from build123d import *

# Parameters (mm, degrees)
F0_R     = 4.175
F0_W     = 52
F0_H     = 52
F0_W_2   = 7
F0_W_3   = 5
F0_H_2   = 50
F0_R_2   = 3.175
F1_DEPTH = 2.5
F2_DEPTH = 10
F3_DEPTH = 10
F4_DEPTH = 10


with BuildPart() as f1:
    # F0 (on Top) → F1 (new body)
    with BuildSketch(Plane.XY):
        with BuildLine():
            Line((-84, -30), (84, -30))
            ThreePointArc((84, -30), (88.2426406871, -28.2426406871), (90, -24))
            Line((90, -24), (90, 24))
            ThreePointArc((90, 24), (88.2426406871, 28.2426406871), (84, 30))
            Line((84, 30), (-84, 30))
            ThreePointArc((-84, 30), (-88.2426406871, 28.2426406871), (-90, 24))
            Line((-90, 24), (-90, -24))
            ThreePointArc((-90, -24), (-88.2426406871, -28.2426406871), (-84, -30))
        make_face()
        with BuildLine():
            ThreePointArc((89, -23), (87.2426406871, -27.2426406871), (83, -29))
            Line((83, -29), (-83, -29))
            ThreePointArc((-83, -29), (-87.2426406871, -27.2426406871), (-89, -23))
            Line((-89, -23), (-89, 23))
            ThreePointArc((-89, 23), (-87.2426406871, 27.2426406871), (-83, 29))
            Line((-83, 29), (83, 29))
            ThreePointArc((83, 29), (87.2426406871, 27.2426406871), (89, 23))
            Line((89, 23), (89, -23))
        make_face(mode=Mode.SUBTRACT)
        with BuildLine():
            Line((-83, -29), (83, -29))
            ThreePointArc((83, -29), (87.2426406871, -27.2426406871), (89, -23))
            Line((89, -23), (89, 23))
            ThreePointArc((89, 23), (87.2426406871, 27.2426406871), (83, 29))
            Line((83, 29), (-83, 29))
            ThreePointArc((-83, 29), (-87.2426406871, 27.2426406871), (-89, 23))
            Line((-89, 23), (-89, -23))
            ThreePointArc((-89, -23), (-87.2426406871, -27.2426406871), (-83, -29))
        make_face()
        with Locations((-82, 0)):
            Circle(F0_R, mode=Mode.SUBTRACT)
        with Locations((-45, 0)):
            Rectangle(F0_W, F0_H, mode=Mode.SUBTRACT)
        with Locations((70, 0)):
            Rectangle(F0_W_2, F0_H, mode=Mode.SUBTRACT)
        with Locations((-45, 0)):
            Rectangle(F0_W, F0_H)
        Polygon((-20, 0), (-20, -25), (-45, -25), (-70, -25), (-70, 0), (-70, 25), (-45, 25), (-20, 25), align=None, mode=Mode.SUBTRACT)
        with Locations((70, 0)):
            Rectangle(F0_W_2, F0_H)
        with Locations((70, 0)):
            Rectangle(F0_W_3, F0_H_2, mode=Mode.SUBTRACT)
        with Locations((70, 0)):
            Rectangle(F0_W_3, F0_H_2)
        with BuildLine():
            Line((-45, -25), (-20, -25))
            Line((-20, -25), (-20, 0))
            ThreePointArc((-20, 0), (-27.3223304703, -17.6776695297), (-45, -25))
        make_face()
        with BuildLine():
            ThreePointArc((-45, 25), (-27.3223304703, 17.6776695297), (-20, 0))
            Line((-20, 0), (-20, 25))
            Line((-20, 25), (-45, 25))
        make_face()
        with BuildLine():
            Line((-70, 25), (-70, 0))
            ThreePointArc((-70, 0), (-62.6776695297, 17.6776695297), (-45, 25))
            Line((-45, 25), (-70, 25))
        make_face()
        with BuildLine():
            Line((-70, -25), (-45, -25))
            ThreePointArc((-45, -25), (-62.6776695297, -17.6776695297), (-70, 0))
            Line((-70, 0), (-70, -25))
        make_face()
        with Locations((-82, 0)):
            Circle(F0_R)
        with Locations((-82, 0)):
            Circle(F0_R_2, mode=Mode.SUBTRACT)
        with Locations((-82, 0)):
            Circle(F0_R_2)
    extrude(amount=F1_DEPTH)

    # F0 (on Top) → F2 (join)
    with BuildSketch(Plane.XY):
        with Locations((-45, 0)):
            Rectangle(F0_W, F0_H)
        Polygon((-20, 0), (-20, -25), (-45, -25), (-70, -25), (-70, 0), (-70, 25), (-45, 25), (-20, 25), align=None, mode=Mode.SUBTRACT)
        with Locations((70, 0)):
            Rectangle(F0_W_2, F0_H)
        with Locations((70, 0)):
            Rectangle(F0_W_3, F0_H_2, mode=Mode.SUBTRACT)
    extrude(amount=F2_DEPTH)

    # F0 (on Top) → F3 (join)
    with BuildSketch(Plane.XY):
        with Locations((-82, 0)):
            Circle(F0_R)
        with Locations((-82, 0)):
            Circle(F0_R_2, mode=Mode.SUBTRACT)
    extrude(amount=F3_DEPTH)

    # F0 (on Top) → F4 (join)
    with BuildSketch(Plane.XY):
        with BuildLine():
            Line((-84, -30), (84, -30))
            ThreePointArc((84, -30), (88.2426406871, -28.2426406871), (90, -24))
            Line((90, -24), (90, 24))
            ThreePointArc((90, 24), (88.2426406871, 28.2426406871), (84, 30))
            Line((84, 30), (-84, 30))
            ThreePointArc((-84, 30), (-88.2426406871, 28.2426406871), (-90, 24))
            Line((-90, 24), (-90, -24))
            ThreePointArc((-90, -24), (-88.2426406871, -28.2426406871), (-84, -30))
        make_face()
        with BuildLine():
            ThreePointArc((89, -23), (87.2426406871, -27.2426406871), (83, -29))
            Line((83, -29), (-83, -29))
            ThreePointArc((-83, -29), (-87.2426406871, -27.2426406871), (-89, -23))
            Line((-89, -23), (-89, 23))
            ThreePointArc((-89, 23), (-87.2426406871, 27.2426406871), (-83, 29))
            Line((-83, 29), (83, 29))
            ThreePointArc((83, 29), (87.2426406871, 27.2426406871), (89, 23))
            Line((89, 23), (89, -23))
        make_face(mode=Mode.SUBTRACT)
    extrude(amount=F4_DEPTH)


solid = f1.part
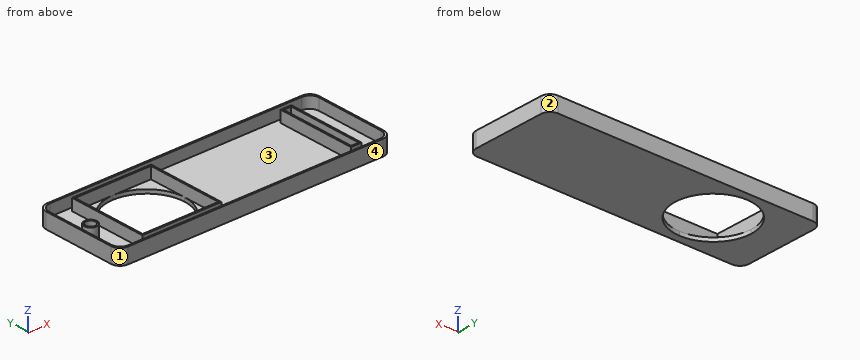
The model under review builds one solid part; all positions refer to its coordinate system, in mm. Face numbers are marked on the shaded views. Round coordinates to 2 decimals unless told otherwise and drop trailing zeros. Loops run counter-clockwise (first coordinate to the right, second up) from the corner with the lowest first, then second, coordinate; pieces in that order, holes last. Notation, with made-up numbers: (17.5, 13) -> (55.5, 13) arc R18 ccw to (55.5, 48) -> close; hole circle Ø6 at (83, 86.5). An arc over 180 degrees is marked (long way). Write item = value, one per line. Start each with the question number.
Item 1: Mouldability with a two-part tool opening along X and no side actions: class the marked faces 1, 2, 3 and 4 as released by +X, released by -X, zero draft, split by the parting line, or undercut.
Item 2: Take a section at B-B on y = 6. Give the boundary of the cut face in (x, z).
Item 3: To check wall thickness, follow L1, parallel to X at y = 21, z = 6.25; L2, parallel to Y at x = -82, z = 6 (3 decimals); L3, parallel to Y at x = -43.5, z = 7. State the ranges of each line that lie inside material, in increasing order.
Item 4: Take a section at D-D on y = -9.5. Give the boundary of the cut face in (x, z).
Item 5: Insertion check: pin 1 (7 mm diameter, centred on x = -81.5, y = -1.5, fed in from +Z); pin 2 (5 mm diameter, centred on x = -24.5, y = -17, fed in from +Z). Each pin has a flat end and moves straight along its axis. Give the tip position at first contact, or say it passes through.
Item 6: Take a section at A-A on z = 5.75. Count the separate pieces of the cut face and the enclosed holes in it, plus the area to 3 significant figures.
Item 7: Take a section at C-C on x = 52.5. Give the boundary of the cut face in (y, z).
Result:
q1.face_1 = released by -X
q1.face_2 = released by +X
q1.face_3 = undercut
q1.face_4 = zero draft
q2.outline = (-90, 0) -> (-69.27, 0) -> (-69.27, 2.5) -> (-70, 2.5) -> (-70, 10) -> (-71, 10) -> (-71, 2.5) -> (-89, 2.5) -> (-89, 10) -> (-90, 10) -> close; (-20.73, 0) -> (90, 0) -> (90, 10) -> (89, 10) -> (89, 2.5) -> (73.5, 2.5) -> (73.5, 10) -> (72.5, 10) -> (72.5, 2.5) -> (67.5, 2.5) -> (67.5, 10) -> (66.5, 10) -> (66.5, 2.5) -> (-19, 2.5) -> (-19, 10) -> (-20, 10) -> (-20, 2.5) -> (-20.73, 2.5) -> close
q3.L1 = -90 to -89, -71 to -70, -20 to -19, 66.5 to 67.5, 72.5 to 73.5, 89 to 90
q3.L2 = -30 to -29, -4.175 to -3.175, 3.175 to 4.175, 29 to 30
q3.L3 = -30 to -29, -26 to -25, 25 to 26, 29 to 30
q4.outline = (-90, 0) -> (-68.12, 0) -> (-68.12, 2.5) -> (-70, 2.5) -> (-70, 10) -> (-71, 10) -> (-71, 2.5) -> (-89, 2.5) -> (-89, 10) -> (-90, 10) -> close; (-21.88, 0) -> (90, 0) -> (90, 10) -> (89, 10) -> (89, 2.5) -> (73.5, 2.5) -> (73.5, 10) -> (72.5, 10) -> (72.5, 2.5) -> (67.5, 2.5) -> (67.5, 10) -> (66.5, 10) -> (66.5, 2.5) -> (-19, 2.5) -> (-19, 10) -> (-20, 10) -> (-20, 2.5) -> (-21.88, 2.5) -> close
q5.pin_1 = 10
q5.pin_2 = 2.5
q6.separate_pieces = 4
q6.enclosed_holes = 4
q6.area = 817 mm²
q7.outline = (-30, 0) -> (30, 0) -> (30, 10) -> (29, 10) -> (29, 2.5) -> (-29, 2.5) -> (-29, 10) -> (-30, 10) -> close
